The listing builds one solid part. Answer for the finished solid, in the listing's coordinates (mm). Face numbers are marked on the shaded views. Round coordinates to 2 decimals unless told otherwise and drop trailing zeros. Loops run counter-clockwise (first coordinate to the right, second up) from the corner with the lowest first, then second, coordinate; pieces in that order, holes last. Notation, with made-up numbers: M 87,19 L 121,19 A15 ccw 121,24 Z; hole C 66.25,25 d3. An arc over 180 degrees is marked long. Put each result on its own line as item: value. Start each with the question number.
(1) Straight lines are drawn through the part: line 1 (X direction, y = -1.25, z = 230.5); line 2 (X direction, y = -6.5, z = 374); line 3 (Z direction, x = 177.8, y = 0.3). For each, find the intervals that lie inside material, in ascending order.
(2) Determine the mould class of the marked faces 1 and 2 for opening direction X: released by +X, released by -X, zero draft, split by the parting line, or undercut.
(3) Section A-A, the plane z = 53.5 is taken. Determine the outline of the cut face in (x, y) (3 decimals), then the cut area to 3 significant figures.
(4) Flat-ended cylindrical pins translate along their axes: P1, Ø1.5, axis at x = -157.5, z = 180.5, coming from the -Y side; P2, Ø5.5, axis at y = -8.31, z = 203.2, coming from the -X side. Find the tip coordinate at first contact, or state that the pin passes through.
(5) Section B-B, the plane x = 32 is taken. Determine the outline of the cut face in (y, z), then the cut area to 3 significant figures.
```python
from build123d import *

# Parameters (mm, degrees)
BASE_FLANGE1_DEPTH = 405.892
FILLET1_R          = 2.54
SKETCH3_R          = 2.4765
CUT_EXTRUDE1_DEPTH = 593.315696883
SKETCH4_R          = 2.4765
CUT_EXTRUDE2_DEPTH = 1.2192


# Sheet-metal steps are written as plain solids
with BuildPart() as part:
    # Sketch1 → Base-Flange1 (new body)
    with BuildSketch(Plane.XY):
        with BuildLine():
            Line((-214.3252, -15.875), (-214.3252, -1.905))
            ThreePointArc((-214.3252, -1.905), (-213.767238418, -0.557961582), (-212.4202, 0))
            Line((-212.4202, 0), (212.4202, 0))
            ThreePointArc((212.4202, 0), (213.767238418, -0.557961582), (214.3252, -1.905))
            Line((214.3252, -1.905), (214.3252, -15.875))
            Line((214.3252, -15.875), (215.5444, -15.875))
            Line((215.5444, -15.875), (215.5444, -1.905))
            ThreePointArc((215.5444, -1.905), (214.629343006, 0.304143006), (212.4202, 1.2192))
            Line((212.4202, 1.2192), (-212.4202, 1.2192))
            ThreePointArc((-212.4202, 1.2192), (-214.629343006, 0.304143006), (-215.5444, -1.905))
            Line((-215.5444, -1.905), (-215.5444, -15.875))
            Line((-215.5444, -15.875), (-214.3252, -15.875))
        make_face()
    extrude(amount=BASE_FLANGE1_DEPTH)

    # Fillet1
    fillet1_edges = [part.edges().sort_by_distance(p)[0] for p in [
        (214.9348, -15.875, 0),
        (214.9348, -15.875, 405.892),
        (-214.9348, -15.875, 405.892),
        (-214.9348, -15.875, 0),
    ]]
    fillet(fillet1_edges, radius=FILLET1_R)

    # Sketch3 → Cut-Extrude1 (cut, through all)
    with BuildSketch(Plane(origin=(215.5444, 0, 0), x_dir=(0, 0, -1), z_dir=(1, 0, 0))):
        with Locations((-393.7, -8.305800148)):
            Circle(SKETCH3_R)
        with Locations((-203.2, -8.305800148)):
            Circle(SKETCH3_R)
        with Locations((-12.7, -8.305800148)):
            Circle(SKETCH3_R)
    extrude(amount=-CUT_EXTRUDE1_DEPTH, mode=Mode.SUBTRACT)

    # Sketch4 → Cut-Extrude2 (cut)
    with BuildSketch(Plane(origin=(0, 1.2192, 0), x_dir=(1, 0, 0), z_dir=(0, 1, 0))):
        with Locations(Location((-177.8, -12.7, 0), (0, 0, 180))):
            Circle(SKETCH4_R)
        with Locations(Location((0, -12.7, 0), (0, 0, 180))):
            Circle(SKETCH4_R)
        with Locations(Location((177.8, -12.7, 0), (0, 0, 180))):
            Circle(SKETCH4_R)
    extrude(amount=-CUT_EXTRUDE2_DEPTH, mode=Mode.SUBTRACT)


solid = part.part
```
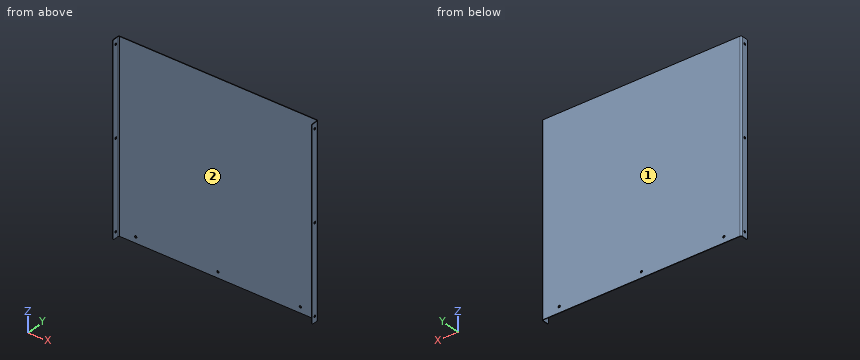
Recorded:
1. line 1: x = -215.47 to -214.21, 214.21 to 215.47
1. line 2: x = -215.54 to -214.33, 214.33 to 215.54
1. line 3: z = 0 to 10.22, 15.18 to 405.89
2. face 1: zero draft
2. face 2: undercut
3. outline: M -215.544,-15.875 L -214.325,-15.875 L -214.325,-1.905 A1.905 cw -212.42,0 L 212.42,0 A1.905 cw 214.325,-1.905 L 214.325,-15.875 L 215.544,-15.875 L 215.544,-1.905 A3.124 ccw 212.42,1.219 L -212.42,1.219 A3.124 ccw -215.544,-1.905 Z
3. area: 562 mm²
4. P1: stops at y = 0
4. P2: stops at x = -215.54
5. outline: M 0,0 L 1.22,0 L 1.22,405.89 L 0,405.89 Z
5. area: 495 mm²
